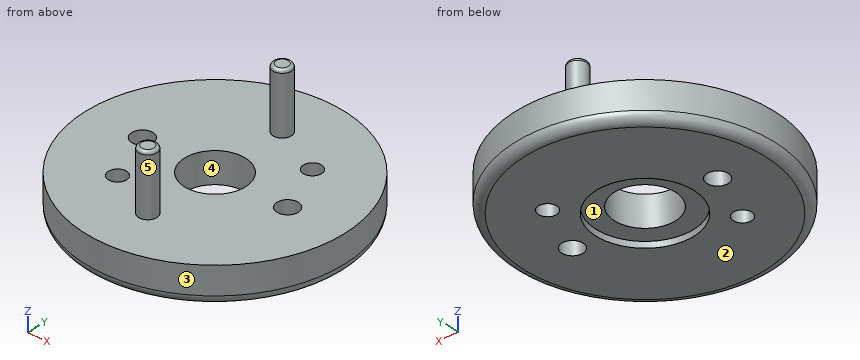
from build123d import *

# Parameters (mm, degrees)
F2_R     = 3
F3_R     = 3.5
F4_DEPTH = 25
F3_R_2   = 3
F5_DEPTH = 20
F6_R     = 1
F7_R     = 3
F8_DEPTH = 25


with BuildPart() as f1:
    # F0 (on Front) → F1 (revolve)
    with BuildSketch(Plane.XZ):
        Polygon((-42.5, 0), (-16, 0), (-16, 2), (-10, 2), (-10, 12), (-42.5, 12), align=None)
    revolve(axis=Axis((0, 0, 19.633664), (0, 0, 1)))

    # F2
    f2_edges = [f1.edges().sort_by_distance(p)[0] for p in [
        (42.5, 0, 0),
    ]]
    fillet(f2_edges, radius=F2_R)

    # F3 (on face) → F4 (cut)
    with BuildSketch(Plane.XY.offset(12)):
        with Locations((-24, 0)):
            Circle(F3_R)
        with Locations((24, 0)):
            Circle(F3_R)
    extrude(amount=-F4_DEPTH, mode=Mode.SUBTRACT)

    # F3 (on face) → F5 (join)
    with BuildSketch(Plane.XY.offset(12)):
        with Locations((0, -25)):
            Circle(F3_R_2)
        with Locations((0, 25)):
            Circle(F3_R_2)
    extrude(amount=F5_DEPTH)

    # F6
    f6_edges = [f1.edges().sort_by_distance(p)[0] for p in [
        (-3, -25, 32),
        (-3, 25, 32),
    ]]
    fillet(f6_edges, radius=F6_R)

    # F7 (on face) → F8 (cut)
    with BuildSketch(Plane.XY.offset(12)):
        with Locations((-17.050904, -17.050904)):
            Circle(F7_R)
        with Locations((17.050904, 17.050904)):
            Circle(F7_R)
    extrude(amount=-F8_DEPTH, mode=Mode.SUBTRACT)


solid = f1.part
Input: part model. Units: mm. Frame: model coordinates. Face numbers are marked on the shaded views. A direction names the side the tool comes from. Give positions to 0.01 mm unless a question says otherwise; leave off trailing zeros. Write each loop counter-clockwise with the first axis right and the second up, starting at its lowest first coordinate (ties: lowest second). Pieces come first, ordered by that corner, then holes. Notation, with made-up numbers: (43.5, 68.25) -> (91.5, 68.25) arc R33 cw to (91.5, 101.25) -> close; hole circle Ø4 at (-27, 59.25). An arc over 180 degrees is marked (long way). Use one line per item in the form item = value. Start each with the question number.
1) Draft query along Y for the marked faces 1, 2 and 3. Return one class per face: pulls with the +Y half, pulls with the -Y half, needs draft (parallel to the pull), parting line crosses it, or undercut.
2) Set-up query: the marked faces 4 and 5. Return all of +Z, -Z, +X, -X, +Y, -Y with unobstructed straight access to the full face (end or side cutting, diameter ignored); none if empty.
3) Pin query (flat end, axial travel): pin 1 (12 mm diameter, centred on y = -22, z = 21.5, fed in from +X); pin 2 (10 mm diameter, centred on x = 12.5, z = 15.5, fed in from +Y); pin 3 (3 mm diameter, centred on x = 1.5, z = 12, fed in from -Y). Return the tip coordinate at first contact, or that it passes through.
4) Section query B-B on z = 15.5. Return the cut outline in (x, y).
5) Section query A-A on x = 0. Return the cut outline in (y, z), then the cut area to 3 significant figures.
6) Ray query, probe 1 along Z at (x, y) = (14.5, 10); probe 2 along Y at (x, z) = (23, 8.5); probe 3 along X at (y, z) = (-2.5, 8.5). Return the intervals inside material, ascending. Write a range as from..to.
Outcome:
q1.face_1 = undercut
q1.face_2 = needs draft
q1.face_3 = parting line crosses it
q2.face_4 = +Z, -Z
q2.face_5 = +Z
q3.pin_1 = 3
q3.pin_2 = 41.55
q3.pin_3 = -42.5
q4.outline = circle Ø6 at (0, -25); circle Ø6 at (0, 25)
q5.outline = (-42.5, 3) arc R3 ccw to (-39.5, 0) -> (-16, 0) -> (-16, 2) -> (-10, 2) -> (-10, 12) -> (-22, 12) -> (-22, 31) arc R1 ccw to (-23, 32) -> (-27, 32) arc R1 ccw to (-28, 31) -> (-28, 12) -> (-42.5, 12) -> close; (10, 2) -> (16, 2) -> (16, 0) -> (39.5, 0) arc R3 ccw to (42.5, 3) -> (42.5, 12) -> (28, 12) -> (28, 31) arc R1 ccw to (27, 32) -> (23, 32) arc R1 ccw to (22, 31) -> (22, 12) -> (10, 12) -> close
q5.area = 991 mm^2
q6.probe_1 = 0..12
q6.probe_2 = -35.74..-3.35, 3.35..35.74
q6.probe_3 = -42.43..-26.45, -21.55..-9.68, 9.68..21.55, 26.45..42.43
